Autodesk Inventor part; units mm, degrees
ref_plane "YZ Plane" through (0, 0, 0) normal (1, 0, 0) x (0, 1, 0)
ref_plane "XZ Plane" through (0, 0, 0) normal (0, 1, 0) x (-1, 0, 0)
ref_plane "XY Plane" through (0, 0, 0) normal (0, 0, 1) x (1, 0, 0)
sketch "Sketch1" plane through (0, 0, 0) normal (0, 1, 0) x (-1, 0, 0)
  arc A0 (9.9875, 99.5) -> (-9.9875, 99.5) centre (0, 100) ccw
  arc A1 (91.1633, 41.1006) -> (81.1758, 58.3994) centre (86.6025, 50) ccw
  arc A2 (81.1758, -58.3994) -> (91.1633, -41.1006) centre (86.6025, -50) ccw
  arc A3 (-9.9875, -99.5) -> (9.9875, -99.5) centre (0, -100) ccw
  arc A4 (-91.1633, -41.1006) -> (-81.1758, -58.3994) centre (-86.6025, -50) ccw
  arc A5 (-81.1758, 58.3994) -> (-91.1633, 41.1006) centre (-86.6025, 50) ccw
  arc A6 (81.1758, 58.3994) -> (9.9875, 99.5) centre (0, 0) ccw
  arc A7 (91.1633, -41.1006) -> (91.1633, 41.1006) centre (0, 0) ccw
  arc A8 (9.9875, -99.5) -> (81.1758, -58.3994) centre (0, 0) ccw
  arc A9 (-81.1758, -58.3994) -> (-9.9875, -99.5) centre (0, 0) ccw
  arc A10 (-9.9875, 99.5) -> (-81.1758, 58.3994) centre (0, 0) ccw
  arc A11 (-91.1633, 41.1006) -> (-91.1633, -41.1006) centre (0, 0) ccw
  circle A12 centre (0, 100) radius 5
  circle A13 centre (86.6025, 50) radius 5
  circle A14 centre (86.6025, -50) radius 5
  circle A15 centre (0, -100) radius 5
  circle A16 centre (-86.6025, -50) radius 5
  circle A17 centre (-86.6025, 50) radius 5
  dimension "d3" = 20
  dimension "d4" = 20
  dimension "d5" = 20
  dimension "d6" = 20
  dimension "d7" = 20
  dimension "d8" = 20
  dimension "d9" = 10
  dimension "d10" = 10
  dimension "d11" = 10
  dimension "d12" = 10
  dimension "d13" = 10
  dimension "d14" = 10
extrude "Extrusion1" add sketch "Sketch1" along normal blind 5
sketch "Sketch2" plane through (0, 5, 0) normal (0, 1, 0) x (1, 0, 0)
  circle A0 centre (0, 0) radius 50
  dimension "d17" = 100
extrude "Extrusion2" cut sketch "Sketch2" against normal blind 2
sketch "Sketch3" plane through (0, 3, 0) normal (0, 1, 0) x (1, 0, 0)
  circle A0 centre (0, 0) radius 2.5
  circle A1 centre (-10, -10) radius 1.5
  circle A2 centre (-10, 10) radius 1.5
  circle A3 centre (10, 10) radius 1.5
  circle A4 centre (10, -10) radius 1.5
  dimension "d20" = 5
  dimension "d29" = 3
  dimension "d30" = 3
  dimension "d31" = 3
  dimension "d32" = 3
extrude "Extrusion3" cut sketch "Sketch3" against normal blind 5
properties part number "Base"
The listing builds one solid part. Answer for the finished solid, in the listing's coordinates (mm). A direction names the side the tool comes from. Give positions to 0.01 mm unless a question says otherwise; leave off trailing zeros. Order: outer loops, then holes, each group sorted by start corner. A loop starts at its lowest first (then second) coordinate and runs counter-clockwise, first axis right, second up. Notation, with made-up numbers: (-27.75, 86) - (1.25, 86) arc R28 ccw to (1.25, 125) - close; hole circle Ø4 at (14, -12.75). An arc over 180 degrees is marked (long way). One line per item, written item: value. Start each with the question number.
1) A cutting plane is placed at B-B on y = 3.75. Give the vertices of the cut face in (x, z).
2) A tool of negligible diameter and unlimited length cuts with its end or side. For faces 4 (the face through (81.833, 2.465, -51.502)), 5 (the face through (-1, 3, 10)), from which of +Z, -Z, +X, -X, +Y, -Y can it reach the whole face along a straight path? Write none if from no direction.
3) Given pin 1 Ø5 at (x, z) = (-10, -10) entering from +Y; pin 2 Ø3 at (x, y) = (45.5, 2) entering from +Z; pin 3 Ø2 at (x, y) = (24, 3) entering from +Z, each flat-ended and moving along its own axis, determine where each tip first touches the part or whether it passes through.
4) Find the intervals of material crossed by L1, parallel to X at y = 1.35, z = -10; L2, parallel to Z at x = 0, y = 3.4; L3, parallel to Z at x = 85, y = 0.7, in increasing order.
5) The mould has two halves that part along X. Classify faces 1 (the face through (1.08, 2.46, 104.88)), 2 (the face through (0, 2, -110)), 3 (the face through (1, 0, -23)): released by +X, released by -X, zero draft, split by the parting line, or undercut.
6) A cutting plane is placed at C-C on x = 87.5. Give the vertices of the cut face in (y, z), then the cut area to 3 significant figures.
7) A cutting plane is placed at D-D on z = -28.5. Give the vertices of the cut face in (x, y).
8) A cutting plane is placed at A-A on x = 0. Give the vertices of the cut face in (y, z), then the cut area to 3 significant figures.
Answer sheet:
1. outline: (-91.16, -41.1) arc R10 ccw (long way) to (-81.18, -58.4) arc R100 ccw to (-9.99, -99.5) arc R10 ccw (long way) to (9.99, -99.5) arc R100 ccw to (81.18, -58.4) arc R10 ccw (long way) to (91.16, -41.1) arc R100 ccw to (91.16, 41.1) arc R10 ccw (long way) to (81.18, 58.4) arc R100 ccw to (9.99, 99.5) arc R10 ccw (long way) to (-9.99, 99.5) arc R100 ccw to (-81.18, 58.4) arc R10 ccw (long way) to (-91.16, 41.1) arc R100 ccw to start; hole circle Ø10 at (-86.6, -50); hole circle Ø10 at (-86.6, 50); hole circle Ø100 at (0, 0); hole circle Ø10 at (0, -100); hole circle Ø10 at (0, 100); hole circle Ø10 at (86.6, -50); hole circle Ø10 at (86.6, 50)
2. face 4: +Y, -Y
2. face 5: +Y
3. pin 1: stops at y = 3
3. pin 2: stops at z = 89.8
3. pin 3: stops at z = 97.32
4. L1: x = -99.5 to -11.5, -8.5 to 8.5, 11.5 to 99.5
4. L2: z = -110 to -105, -95 to -50, 50 to 95, 105 to 110
4. L3: z = -59.87 to -54.74, -45.26 to 45.26, 54.74 to 59.87
5. face 1: undercut
5. face 2: split by the parting line
5. face 3: zero draft
6. outline: (0, -59.96) - (5, -59.96) - (5, -54.92) - (0, -54.92) - close; (0, -45.08) - (5, -45.08) - (5, 45.08) - (0, 45.08) - close; (0, 54.92) - (5, 54.92) - (5, 59.96) - (0, 59.96) - close
6. area: 501 mm2
7. outline: (-95.85, 0) - (95.85, 0) - (95.85, 5) - (41.08, 5) - (41.08, 3) - (-41.08, 3) - (-41.08, 5) - (-95.85, 5) - close
8. outline: (0, -110) - (5, -110) - (5, -105) - (0, -105) - close; (0, -95) - (5, -95) - (5, -50) - (3, -50) - (3, -2.5) - (0, -2.5) - close; (0, 2.5) - (3, 2.5) - (3, 50) - (5, 50) - (5, 95) - (0, 95) - close; (0, 105) - (5, 105) - (5, 110) - (0, 110) - close
8. area: 785 mm2
